Design review of the part built by this model. Coordinates are the model's own, in mm. Coordinates: 2 decimals unless noted, no trailing zeros. Loops run counter-clockwise (first coordinate to the right, second up) from the corner with the lowest first, then second, coordinate; pieces in that order, holes last.
Q1. Add section C-C on x = 38.1. Give the boundary of the cut face in (y, z) (3 decimals), and give its area (3 significant figures).
Q2. Add section A-A on x = 63.5. Give the boundary of the cut face in (y, z) (3 decimals), and give its area (3 significant figures).
Q3. Wall thickness on probe 1 along X at (y, z) = (1.8, 63.5); probe 2 along Z at (x, y) = (38.1, 1.25); probe 3 along X at (y, z) = (0.8, 38.1): over which ranges is each line inside the solid? List them lowest first.
Q4. For P1, Ø3.5, axis at x = 63.5, z = 50.8, coming from the -Y side, flat-tipped, find the tip position at first contact; note if it passes through.
Q5. Add section D-D on z = 63.5. Give the boundary of the cut face in (x, y) (3 decimals), and give its area (3 significant figures).
Q6. Add section B-B on z = 88.9. Give the boundary of the cut face in (x, y) (3 decimals).
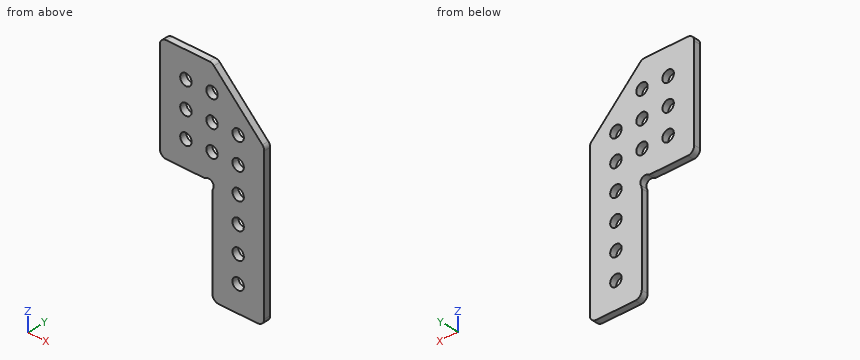
Autodesk Fusion 360 part; units mm, degrees
sketch "Sketch1" plane through (0, 0, 0) normal (0, 1, 0) x (1, 0, 0)
  line L0 (0, 0) -> (0, -76.2)
  line L1 (0, -76.2) -> (76.2, -76.2)
  line L2 (76.2, -76.2) -> (76.2, 0)
  line L3 (76.2, 0) -> (50.927, 0)
  line L4 (50.927, 0) -> (50.927, -50.8)
  line L5 (50.927, -50.8) -> (25.273, -50.8)
  line L6 (25.273, -50.8) -> (25.273, 0)
  line L7 (25.273, 0) -> (0, 0)
  line L8 (12.7, 0) -> (12.7, -76.2) construction
  line L9 (38.1, -50.8) -> (38.1, -76.2) construction
  circle A0 centre (26.9568, -49.1162) radius 2.3813
  line L10 (26.9568, -49.1162) -> (26.9568, -50.8) construction
  line L11 (26.9568, -49.1162) -> (25.273, -49.1162) construction
  circle A1 centre (12.7, -12.7) radius 2.7781
  circle A2 centre (12.7, -25.4) radius 2.7781
  line L12 (12.7, -12.7) -> (12.7, -88.9) construction
  circle A3 centre (12.7, -38.1) radius 2.7781
  line L13 (12.7, -25.4) -> (12.7, -101.6) construction
  circle A4 centre (12.7, -50.8) radius 2.7781
  line L14 (12.7, -38.1) -> (12.7, -114.3) construction
  circle A5 centre (12.7, -63.5) radius 2.7781
  line L15 (12.7, -50.8) -> (12.7, -127) construction
  circle A6 centre (63.5, -38.1) radius 2.7781
  circle A7 centre (63.5, -50.8) radius 2.7781
  circle A8 centre (63.5, -63.5) radius 2.7781
  circle A9 centre (63.5, -25.4) radius 2.7781
  circle A10 centre (63.5, -12.7) radius 2.7781
  circle A11 centre (49.2432, -49.1162) radius 2.3813
  circle A12 centre (38.1, -63.5) radius 2.7781
  line L16 (0, -76.2) -> (25.4, -101.6)
  line L17 (25.4, -101.6) -> (50.8, -101.6)
  line L18 (50.8, -101.6) -> (76.2, -76.2)
  circle A13 centre (38.1, -76.2) radius 2.7781
  circle A14 centre (38.1, -88.9) radius 2.7781
  circle A15 centre (25.4, -63.5) radius 2.7781
  circle A16 centre (25.4, -76.2) radius 2.7781
  circle A17 centre (25.4, -88.9) radius 2.7781
  circle A18 centre (12.7, -76.2) radius 2.7781
  circle A19 centre (50.8, -63.5) radius 2.7781
  circle A20 centre (50.8, -76.2) radius 2.7781
  circle A21 centre (50.8, -88.9) radius 2.7781
  circle A22 centre (63.5, -76.2) radius 2.7781
  dimension "d1" = 76.2
  dimension "d3" = 25.654
  dimension "d4" = 50.8
  dimension "d6" = 76.2
  dimension "d7" = 12.7
  dimension "d8" = 4.7625
  dimension "d9" = 5.5563
  dimension "d10" = 12.7
  dimension "d13" = 0
  dimension "d14" = -50.8
  dimension "d17" = 25.4
  dimension "d18" = 0
  dimension "d25" = 25.4
  dimension "d26" = 25.4
  dimension "d29" = 25.4
  dimension "d30" = 0
  dimension "d33" = 12.7
  dimension "d34" = 0
  dimension "d37" = 0
  dimension "d38" = -25.4
  dimension "d41" = 0
  dimension "d42" = -12.7
extrude "Extrude1" add sketch "Sketch1" along normal blind 3.175 contours L0 L1 L2 L3 L4 L5 L6 L7 A0 A11 A13 A16 A18 A20 A22 | L1 L16 L17 L18 A13 A16 A18 A20 A22 | L1 A18 | L1 A18 | L6 A0 | L5 A0 | L1 A16 | L1 A16 | A1 | A2 | A3 | A4 | A5 | A15 | A17 makes body 1
ref_plane "WorkPlane1" through (25.4, 1.5875, 38.1) normal (-1, 0, 0) x (0, 0, 1)
split "Split1" by plane through (25.4, 1.5875, 38.1) normal (-1, 0, 0) bodies 1 makes body 2 at (8.4243, 0, 42.3333)
delete_body "RemoveBody1" bodies 2
fillet "Fillet1" radius 3.175 6 edges at (50.927, 1.5875, 0) (76.2, 1.5875, 0) (50.8, 1.5875, 101.6) (76.2, 1.5875, 76.2) (25.4, 1.5875, 101.6) (25.4, 1.5875, 50.8) on bodies 1
fillet "Fillet1" radius 3.175 2 edges at (47.5594, 1.5875, 50.8) (50.927, 1.5875, 47.4324) on bodies 1
sketch "DXF" plane through (0, 0, 0) normal (0, -1, 0) x (1, 0, 0)
  arc A0 (51.3255, 47.9611) -> (50.927, 46.421) centre (54.102, 46.421) ccw
  line L0 (50.927, 46.421) -> (50.927, 3.175)
  arc A1 (50.927, 3.175) -> (54.102, 0) centre (54.102, 3.175) ccw
  line L1 (54.102, 0) -> (73.025, 0)
  arc A2 (73.025, 0) -> (76.2, 3.175) centre (73.025, 3.175) ccw
  line L2 (76.2, 3.175) -> (76.2, 74.8849)
  arc A3 (76.2, 74.8849) -> (75.2701, 77.1299) centre (73.025, 74.8849) ccw
  line L3 (75.2701, 77.1299) -> (51.7299, 100.6701)
  arc A4 (51.7299, 100.6701) -> (49.4849, 101.6) centre (49.4849, 98.425) ccw
  line L4 (49.4849, 101.6) -> (28.575, 101.6)
  arc A5 (28.575, 101.6) -> (25.4, 98.425) centre (28.575, 98.425) ccw
  line L5 (25.4, 98.425) -> (25.4, 53.975)
  arc A6 (25.4, 53.975) -> (28.575, 50.8) centre (28.575, 53.975) ccw
  line L6 (28.575, 50.8) -> (46.548, 50.8)
  arc A7 (46.548, 50.8) -> (48.0881, 51.1985) centre (46.548, 53.975) ccw
  arc A8 (51.3255, 47.9611) -> (48.0881, 51.1985) centre (49.2432, 49.1162) ccw
  circle A9 centre (50.8, 88.9) radius 2.7781
  circle A10 centre (50.8, 63.5) radius 2.7781
  circle A11 centre (63.5, 25.4) radius 2.7781
  circle A12 centre (38.1, 88.9) radius 2.7781
  circle A13 centre (38.1, 63.5) radius 2.7781
  circle A14 centre (63.5, 50.8) radius 2.7781
  circle A15 centre (63.5, 63.5) radius 2.7781
  circle A16 centre (63.5, 38.1) radius 2.7781
  circle A17 centre (50.8, 76.2) radius 2.7781
  circle A18 centre (38.1, 76.2) radius 2.7781
  circle A19 centre (63.5, 12.7) radius 2.7781
  circle A20 centre (63.5, 76.2) radius 2.7781
equation "TOLERANCE = 0.01 in"
equation "d3 = 1 in + TOLERANCE"
equation "d9 = ( 7 / 32 ) * 1 in"
Entries:
1. outline: (0, 50.8) - (3.175, 50.8) - (3.175, 60.722) - (0, 60.722) - close; (0, 66.278) - (3.175, 66.278) - (3.175, 73.422) - (0, 73.422) - close; (0, 78.978) - (3.175, 78.978) - (3.175, 86.122) - (0, 86.122) - close; (0, 91.678) - (3.175, 91.678) - (3.175, 101.6) - (0, 101.6) - close
1. area: 108 mm2
2. outline: (0, 0) - (3.175, 0) - (3.175, 9.922) - (0, 9.922) - close; (0, 15.478) - (3.175, 15.478) - (3.175, 22.622) - (0, 22.622) - close; (0, 28.178) - (3.175, 28.178) - (3.175, 35.322) - (0, 35.322) - close; (0, 40.878) - (3.175, 40.878) - (3.175, 48.022) - (0, 48.022) - close; (0, 53.578) - (3.175, 53.578) - (3.175, 60.722) - (0, 60.722) - close; (0, 66.278) - (3.175, 66.278) - (3.175, 73.422) - (0, 73.422) - close; (0, 78.978) - (3.175, 78.978) - (3.175, 88.9) - (0, 88.9) - close
2. area: 176 mm2
3. probe 1: x = 25.4 to 35.32, 40.88 to 48.02, 53.58 to 60.72, 66.28 to 76.2
3. probe 2: z = 50.8 to 60.72, 66.28 to 73.42, 78.98 to 86.12, 91.68 to 101.6
3. probe 3: x = 50.93 to 60.72, 66.28 to 76.2
4. P1: passes through
5. outline: (25.4, 0) - (35.322, 0) - (35.322, 3.175) - (25.4, 3.175) - close; (40.878, 0) - (48.022, 0) - (48.022, 3.175) - (40.878, 3.175) - close; (53.578, 0) - (60.722, 0) - (60.722, 3.175) - (53.578, 3.175) - close; (66.278, 0) - (76.2, 0) - (76.2, 3.175) - (66.278, 3.175) - close
5. area: 108 mm2
6. outline: (25.4, 0) - (35.322, 0) - (35.322, 3.175) - (25.4, 3.175) - close; (40.878, 0) - (48.022, 0) - (48.022, 3.175) - (40.878, 3.175) - close; (53.578, 0) - (63.5, 0) - (63.5, 3.175) - (53.578, 3.175) - close
